Autodesk Inventor part; units mm, degrees
ref_plane "YZ Plane" through (0, 0, 0) normal (1, 0, 0) x (0, 1, 0)
ref_plane "XZ Plane" through (0, 0, 0) normal (0, 1, 0) x (-1, 0, 0)
ref_plane "XY Plane" through (0, 0, 0) normal (0, 0, 1) x (1, 0, 0)
sketch "Sketch1" plane through (0, 0, 0) normal (0, 1, 0) x (-1, 0, 0)
  line L0 (0, 0) -> (9.91, 0)
  line L1 (9.91, 0) -> (9.91, -19.22)
  line L2 (9.91, -19.22) -> (0, -19.22)
  line L3 (0, -19.22) -> (0, 0)
  dimension "d0" = 19.22
  dimension "d1" = 9.91
extrude "Extrusion1" add sketch "Sketch1" along normal blind 258.6
sketch "Sketch2" plane through (0, 0, 0) normal (0, -1, 0) x (1, 0, 0)
  line L0 (0, -1.7) -> (-7, -1.7)
  line L1 (-7, -1.7) -> (-7, -5.84)
  line L2 (-7, -5.84) -> (0, -5.84)
  line L3 (0, -5.84) -> (0, -1.7)
  line L4 (0, 0) -> (-9.91, 0)
  line L5 (0, -19.22) -> (0, 0)
  dimension "d31" = 1.7
  dimension "d32" = 4.14
  dimension "d33" = 7
extrude "Extrusion2" cut sketch "Sketch2" against normal through all
sketch "Sketch3" plane through (0, 0, 0) normal (0, -1, 0) x (1, 0, 0)
  line L0 (0, -7.54) -> (-7, -7.54)
  line L1 (-7, -7.54) -> (-7, -11.68)
  line L2 (-7, -11.68) -> (0, -11.68)
  line L3 (0, -11.68) -> (0, -7.54)
  line L4 (0, -5.84) -> (-7, -5.84)
  line L5 (-7, -5.84) -> (-7, -1.7)
  point P0 (0, 0)
  dimension "d39" = 1.7
  dimension "d40" = 4.14
extrude "Extrusion3" cut sketch "Sketch3" against normal through all
sketch "Sketch4" plane through (0, 0, 0) normal (0, -1, 0) x (1, 0, 0)
  line L0 (0, -13.38) -> (-7, -13.38)
  line L1 (-7, -13.38) -> (-7, -17.52)
  line L2 (-7, -17.52) -> (0, -17.52)
  line L3 (0, -17.52) -> (0, -13.38)
  line L4 (0, -11.68) -> (-7, -11.68)
  line L5 (-7, -11.68) -> (-7, -7.54)
  point P0 (0, 0)
  dimension "d43" = 1.7
  dimension "d44" = 4.14
extrude "Extrusion4" cut sketch "Sketch4" against normal through all
hole "Hole7" at (0, 3, -6.69) direction (-1, 0, 0) diameter 2.9 end through all counterbore diameter 6.5 counterbore depth 7
hole "Hole8" at (0, 143.4, -6.69) direction (-1, 0, 0) diameter 2.9 end through all counterbore diameter 6.5 counterbore depth 7
sketch "Sketch5" plane through (0, 0, 0) normal (1, 0, 0) x (0, 0, -1)
  line L0 (0, 0) -> (0, 258.6)
  line L1 (13.38, 0) -> (13.38, 258.6)
  line L2 (0, 258.6) -> (13.38, 258.6)
  line L3 (13.38, 258.6) -> (13.38, 241.6)
  line L4 (13.38, 241.6) -> (0, 241.6)
  line L5 (0, 241.6) -> (0, 258.6)
  point P0 (13.38, 146.5369)
  point P1 (13.38, 6.1369)
  dimension "d128" = 17
extrude "Extrusion5" cut sketch "Sketch5" against normal up to surface (7 mm away)
hole "Hole13" at (-7, 255.6, -6.69) direction (-1, 0, 0) diameter 2.9 end through all
sketch "Sketch6" plane through (-9.91, 0, -19.22) normal (-1, 0, 0) x (0, 0, 1)
  line L0 (0, 0) -> (0, 258.6)
  line L1 (19.22, 0) -> (19.22, 258.6)
  line L2 (0, 112.4) -> (19.22, 112.4)
  line L3 (19.22, 112.4) -> (19.22, 85)
  line L4 (19.22, 85) -> (0, 85)
  line L5 (0, 85) -> (0, 112.4)
  line L6 (19.22, 0) -> (0, 0)
  dimension "d149" = 85
  dimension "d150" = 112.4
extrude "Extrusion6" cut sketch "Sketch6" against normal blind 1.45 contours L0 L2 L1 L4
sketch "Sketch7" plane through (-9.91, 258.6, -19.22) normal (-1, 0, 0) x (0, 0, 1)
  line L0 (0, -258.6) -> (0, 0)
  line L1 (19.22, -258.6) -> (19.22, -17)
  line L2 (0, -126.6) -> (19.22, -126.6)
  line L3 (19.22, -126.6) -> (19.22, -144.2)
  line L4 (19.22, -144.2) -> (0, -144.2)
  line L5 (0, -144.2) -> (0, -126.6)
  line L6 (19.22, -258.6) -> (0, -258.6)
  dimension "d153" = 132
  dimension "d154" = 114.4
extrude "Extrusion7" cut sketch "Sketch7" against normal blind 2.65 contours L0 L2 L1 L4
sketch "Sketch8" plane through (-9.91, 258.6, -19.22) normal (-1, 0, 0) x (0, 0, 1)
  line L0 (0, -258.6) -> (0, 0)
  line L1 (19.22, -258.6) -> (19.22, -17)
  line L2 (0, -6.2) -> (19.22, -6.2)
  line L3 (19.22, -6.2) -> (19.22, -33.6)
  line L4 (19.22, -33.6) -> (0, -33.6)
  line L5 (0, -33.6) -> (0, -6.2)
  line L6 (19.22, -258.6) -> (0, -258.6)
  dimension "d157" = 225
  dimension "d158" = 252.4
extrude "Extrusion8" cut sketch "Sketch8" against normal blind 1.45 contours L0 L2 L3 L1 L4
properties part number "6089-110_FF_left_heatsink"
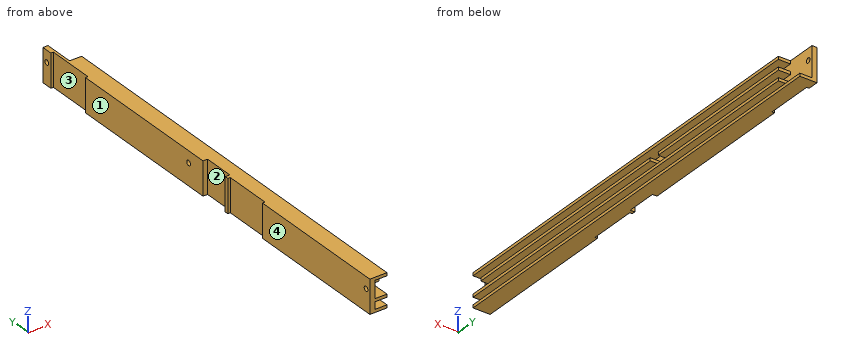
Here's how the part is built. I have some questions about the finished solid (model axes, mm). Face numbers are marked on the shaded views. A direction names the side the tool comes from. Round coordinates to 2 decimals unless told otherwise and drop trailing zeros. Write each loop counter-clockwise with the first axis right and the second up, starting at its lowest first coordinate (ties: lowest second). Pieces come first, ordered by that corner, then holes.
1. Suppose I cut it at B-B (y = 45). List the corners of the cut face in (x, z) for me.
2. Will these pins go through, and if not, where does the flat tip stop? pin 1 Ø0.5 at (x, z) = (-2, -1) entering from +Y; pin 2 Ø4 at (y, z) = (255.6, -6.69) entering from +X.
3. If we mould it in two halves opening along Y, with no side actions, what happens to the marked faces 3 and 4? For each: released by +Y, released by -Y, zero draft, split by the parting line, or undercut.
4. For the marked faces 1 and 2, which set-ups out of +Z, -Z, +X, -X, +Y, -Y let a thin tool reach every point of the face, with its end or its side?
5. Suppose I cut it at A-A (x = -3.75). List the corners of the cut face in (y, z) for me, and give its area (3 significant figures).
6. I need wall thicknesses on L1, parallel to Y at x = -8.15, z = -6.69; L2, parallel to Z at x = -6.5, y = 91.5; L3, parallel to Y at x = -8.5, z = -14.25. Which ranges of each line are inside material? Lowest first, please.
Answer sheet:
1. outline: (-9.91, -19.22) - (0, -19.22) - (0, -17.52) - (-7, -17.52) - (-7, -13.38) - (0, -13.38) - (0, -11.68) - (-7, -11.68) - (-7, -7.54) - (0, -7.54) - (0, -5.84) - (-7, -5.84) - (-7, -1.7) - (0, -1.7) - (0, 0) - (-9.91, 0) - close
2. pin 1: stops at y = 241.6
2. pin 2: stops at x = -7
3. face 3: undercut
3. face 4: zero draft
4. face 1: +Z, -Z, -X, +Y, -Y
4. face 2: +Z, -Z, -X
5. outline: (0, -19.22) - (258.6, -19.22) - (258.6, -17.52) - (0, -17.52) - close; (0, -13.38) - (241.6, -13.38) - (241.6, -11.68) - (0, -11.68) - close; (0, -1.7) - (241.6, -1.7) - (241.6, 0) - (0, 0) - close; (6.14, -7.54) - (140.26, -7.54) arc R3.25 cw to (140.26, -5.84) - (6.14, -5.84) arc R3.25 cw to start; (146.54, -7.54) - (241.6, -7.54) - (241.6, -5.84) - (146.54, -5.84) arc R3.25 cw to start
5. area: 1,650 mm2
6. L1: y = 0 to 1.55, 4.45 to 114.4, 132 to 141.95, 144.85 to 254.15, 257.05 to 258.6
6. L2: z = -19.22 to -17.52, -13.38 to -11.68, -7.54 to -5.84, -1.7 to 0
6. L3: y = 0 to 85, 112.4 to 114.4, 132 to 225, 252.4 to 258.6
